from build123d import *

# Parameters (mm, degrees)
ESQUISSE1_W             = 15
ESQUISSE1_H             = 9.5
BOSS_EXTRU_1_DEPTH      = 0.3
ESQUISSE2_W             = 5
ESQUISSE2_H             = 5
BOSS_EXTRU_2_DEPTH      = 1.6
ESQUISSE3_R             = 2
ENL_V_MAT_EXTRU_1_DEPTH = 0.3
BOSS_EXTRU_3_DEPTH      = 0.2
CONG_1_R                = 0.5
ENL_V_MAT_EXTRU_2_DEPTH = 0.05
ESQUISSE6_W             = 1
ESQUISSE6_H             = 2
BOSS_EXTRU_4_DEPTH      = 1


with BuildPart() as part:
    # Esquisse1 → Boss.-Extru.1 (new body)
    with BuildSketch(Plane.XY):
        with Locations((7.5, 4.75)):
            Rectangle(ESQUISSE1_W, ESQUISSE1_H)
    extrude(amount=BOSS_EXTRU_1_DEPTH)

    # Esquisse2 → Boss.-Extru.2 (add)
    with BuildSketch(Plane.XY.offset(0.3)):
        with Locations((7.5, 4.75)):
            Rectangle(ESQUISSE2_W, ESQUISSE2_H)
    extrude(amount=BOSS_EXTRU_2_DEPTH)

    # Esquisse3 → Enlèv. mat.-Extru.1 (cut)
    with BuildSketch(Plane.XY.offset(1.9)):
        with Locations((7.5, 4.75)):
            Circle(ESQUISSE3_R)
        Polygon((9.292893219, 7.25), (10, 6.542893219), (10, 7.25), align=None)
    extrude(amount=-ENL_V_MAT_EXTRU_1_DEPTH, mode=Mode.SUBTRACT)

    # Esquisse4 → Boss.-Extru.3 (add)
    with BuildSketch(Plane.XY.offset(0.3)):
        with BuildLine():
            Line((8.875, 8.263238259), (8.625, 8.263238259))
            ThreePointArc((8.625, 8.263238259), (8.271446609, 8.11679165), (8.125, 7.763238259))
            Line((8.125, 7.763238259), (8.125, 7.25))
            Line((8.125, 7.25), (9.375, 7.25))
            Line((9.375, 7.25), (9.375, 7.763238259))
            ThreePointArc((9.375, 7.763238259), (9.228553391, 8.11679165), (8.875, 8.263238259))
        make_face()
        with BuildLine():
            Line((5.625, 7.25), (6.875, 7.25))
            Line((6.875, 7.25), (6.875, 7.763238259))
            ThreePointArc((6.875, 7.763238259), (6.728553391, 8.11679165), (6.375, 8.263238259))
            Line((6.375, 8.263238259), (6.125, 8.263238259))
            ThreePointArc((6.125, 8.263238259), (5.771446609, 8.11679165), (5.625, 7.763238259))
            Line((5.625, 7.763238259), (5.625, 7.25))
        make_face()
        with BuildLine():
            Line((9.375, 2.25), (9.375, 1.736761741))
            ThreePointArc((9.375, 1.736761741), (9.228553391, 1.38320835), (8.875, 1.236761741))
            Line((8.875, 1.236761741), (8.625, 1.236761741))
            ThreePointArc((8.625, 1.236761741), (8.271446609, 1.38320835), (8.125, 1.736761741))
            Line((8.125, 1.736761741), (8.125, 2.25))
            Line((8.125, 2.25), (9.375, 2.25))
        make_face()
        with BuildLine():
            Line((6.125, 1.236761741), (6.375, 1.236761741))
            ThreePointArc((6.375, 1.236761741), (6.728553391, 1.38320835), (6.875, 1.736761741))
            Line((6.875, 1.736761741), (6.875, 2.25))
            Line((6.875, 2.25), (5.625, 2.25))
            Line((5.625, 2.25), (5.625, 1.736761741))
            ThreePointArc((5.625, 1.736761741), (5.771446609, 1.38320835), (6.125, 1.236761741))
        make_face()
    extrude(amount=BOSS_EXTRU_3_DEPTH)

    # Congé1
    # the kernel refuses this fillet: 0.5 mm, written as the material it takes off along each edge
    with BuildSketch(Plane(origin=(8.125, 1.736761741, 0.5), x_dir=(2.6165736243852198e-11, 0, -1.0), z_dir=(0, 1, 0)), Plane(origin=(9.375, 2.25, 0.5), x_dir=(-2.6165736243852198e-11, 0, -1.0), z_dir=(0, -1, 0))) as cong_1_piece_1:
        with BuildLine():
            CenterArc((0.5, -0.4), CONG_1_R, 126.869897647, 53.130102355)
            Line((0, -0.4), (-0.01, -0.4))
            Line((-0.01, -0.4), (-0.01, 0))
            Line((-0.01, 0), (0, 0.01))
            ThreePointArc((0, 0.01), (0.1, 0.01), (0.194, 0.008))
            Line((0.194, 0.008), (0.2, 0))
        make_face()
    extrude(amount=0.513238259, mode=Mode.SUBTRACT)
    with BuildSketch(Plane(origin=(8.625, 1.736761741, 0.5), x_dir=(0, -1, 0), z_dir=(1, 0, 0))) as cong_1_piece_2:
        with BuildLine():
            CenterArc((0.1, 0.5), CONG_1_R, 270, 53.130102355)
            Line((0.1, 0), (0.1, -0.01))
            Line((0.1, -0.01), (0.5, -0.01))
            Line((0.5, -0.01), (0.51, 0))
            ThreePointArc((0.51, 0), (0.51, 0.1), (0.508, 0.194))
            Line((0.508, 0.194), (0.5, 0.2))
        make_face()
    revolve(axis=Axis((8.625, 1.736761741, 0.5), (0, 0, -1)), revolution_arc=90, mode=Mode.SUBTRACT)
    with BuildSketch(Plane(origin=(8.875, 1.236761741, 0.5), x_dir=(0, 2.6109114869598534e-11, -1.0), z_dir=(-1, 0, 0))) as cong_1_piece_3:
        with BuildLine():
            CenterArc((0.5, -0.4), CONG_1_R, 126.869897647, 53.130102355)
            Line((0, -0.4), (-0.01, -0.4))
            Line((-0.01, -0.4), (-0.01, 0))
            Line((-0.01, 0), (0, 0.01))
            ThreePointArc((0, 0.01), (0.1, 0.01), (0.194, 0.008))
            Line((0.194, 0.008), (0.2, 0))
        make_face()
    extrude(amount=0.25, mode=Mode.SUBTRACT)
    with BuildSketch(Plane(origin=(5.625, 2.25, 0.5), x_dir=(2.6059154833492393e-11, 0, -1.0), z_dir=(0, -1, 0)), Plane(origin=(6.875, 1.736761741, 0.5), x_dir=(-2.6112445538672294e-11, 0, -1.0), z_dir=(0, 1, 0)), Plane(origin=(6.875, 7.25, 0.5), x_dir=(-2.6112445538672294e-11, 0, -1.0), z_dir=(0, 1, 0)), Plane(origin=(5.625, 7.763238259, 0.5), x_dir=(2.6059154833492393e-11, 0, -1.0), z_dir=(0, -1, 0)), Plane(origin=(9.375, 7.25, 0.5), x_dir=(-2.6165736243852198e-11, 0, -1.0), z_dir=(0, 1, 0)), Plane(origin=(8.125, 7.763238259, 0.5), x_dir=(2.6165736243852198e-11, 0, -1.0), z_dir=(0, -1, 0))) as cong_1_piece_4:
        with BuildLine():
            CenterArc((0.5, 0.4), CONG_1_R, 179.999999999, 53.130102355)
            Line((0, 0.4), (-0.01, 0.4))
            Line((-0.01, 0.4), (-0.01, 0))
            Line((-0.01, 0), (0, -0.01))
            ThreePointArc((0, -0.01), (0.1, -0.01), (0.194, -0.008))
            Line((0.194, -0.008), (0.2, 0))
        make_face()
    extrude(amount=0.513238259, mode=Mode.SUBTRACT)
    with BuildSketch(Plane(origin=(6.125, 1.736761741, 0.5), x_dir=(-1, 0, 0), z_dir=(0, 1, 0))) as cong_1_piece_5:
        with BuildLine():
            CenterArc((0.1, -0.5), CONG_1_R, 36.869897645, 53.130102355)
            Line((0.1, 0), (0.1, 0.01))
            Line((0.1, 0.01), (0.5, 0.01))
            Line((0.5, 0.01), (0.51, 0))
            ThreePointArc((0.51, 0), (0.51, -0.1), (0.508, -0.194))
            Line((0.508, -0.194), (0.5, -0.2))
        make_face()
    revolve(axis=Axis((6.125, 1.736761741, 0.5), (0, 0, 1)), revolution_arc=90, mode=Mode.SUBTRACT)
    with BuildSketch(Plane(origin=(6.125, 1.236761741, 0.5), x_dir=(0, 2.6109114869598534e-11, -1.0), z_dir=(1, 0, 0)), Plane(origin=(6.375, 8.263238259, 0.5), x_dir=(0, -2.6112445538672342e-11, -1.0), z_dir=(-1, 0, 0)), Plane(origin=(8.875, 8.263238259, 0.5), x_dir=(0, -2.6112445538672342e-11, -1.0), z_dir=(-1, 0, 0))) as cong_1_piece_6:
        with BuildLine():
            CenterArc((0.5, 0.4), CONG_1_R, 179.999999999, 53.130102355)
            Line((0, 0.4), (-0.01, 0.4))
            Line((-0.01, 0.4), (-0.01, 0))
            Line((-0.01, 0), (0, -0.01))
            ThreePointArc((0, -0.01), (0.1, -0.01), (0.194, -0.008))
            Line((0.194, -0.008), (0.2, 0))
        make_face()
    extrude(amount=0.25, mode=Mode.SUBTRACT)
    with BuildSketch(Plane(origin=(6.125, 7.763238259, 0.5), x_dir=(0, 1, 0), z_dir=(1, 0, 0))) as cong_1_piece_7:
        with BuildLine():
            CenterArc((0.1, -0.5), CONG_1_R, 36.869897645, 53.130102355)
            Line((0.1, 0), (0.1, 0.01))
            Line((0.1, 0.01), (0.5, 0.01))
            Line((0.5, 0.01), (0.51, 0))
            ThreePointArc((0.51, 0), (0.51, -0.1), (0.508, -0.194))
            Line((0.508, -0.194), (0.5, -0.2))
        make_face()
    revolve(axis=Axis((6.125, 7.763238259, 0.5), (0, 0, 1)), revolution_arc=90, mode=Mode.SUBTRACT)
    with BuildSketch(Plane(origin=(8.875, 7.763238259, 0.5), x_dir=(1, 0, 0), z_dir=(0, -1, 0))) as cong_1_piece_8:
        with BuildLine():
            CenterArc((0.1, -0.5), CONG_1_R, 36.869897645, 53.130102355)
            Line((0.1, 0), (0.1, 0.01))
            Line((0.1, 0.01), (0.5, 0.01))
            Line((0.5, 0.01), (0.51, 0))
            ThreePointArc((0.51, 0), (0.51, -0.1), (0.508, -0.194))
            Line((0.508, -0.194), (0.5, -0.2))
        make_face()
    revolve(axis=Axis((8.875, 7.763238259, 0.5), (0, 0, 1)), revolution_arc=90, mode=Mode.SUBTRACT)
    with BuildSketch(Plane(origin=(8.875, 1.736761741, 0.5), x_dir=(1, 0, 0), z_dir=(0, 1, 0))) as cong_1_piece_9:
        with BuildLine():
            CenterArc((0.1, 0.5), CONG_1_R, 270, 53.130102355)
            Line((0.1, 0), (0.1, -0.01))
            Line((0.1, -0.01), (0.5, -0.01))
            Line((0.5, -0.01), (0.51, 0))
            ThreePointArc((0.51, 0), (0.51, 0.1), (0.508, 0.194))
            Line((0.508, 0.194), (0.5, 0.2))
        make_face()
    revolve(axis=Axis((8.875, 1.736761741, 0.5), (0, 0, -1)), revolution_arc=90, mode=Mode.SUBTRACT)
    with BuildSketch(Plane(origin=(6.375, 1.736761741, 0.5), x_dir=(0, -1, 0), z_dir=(-1, 0, 0))) as cong_1_piece_10:
        with BuildLine():
            CenterArc((0.1, -0.5), CONG_1_R, 36.869897645, 53.130102355)
            Line((0.1, 0), (0.1, 0.01))
            Line((0.1, 0.01), (0.5, 0.01))
            Line((0.5, 0.01), (0.51, 0))
            ThreePointArc((0.51, 0), (0.51, -0.1), (0.508, -0.194))
            Line((0.508, -0.194), (0.5, -0.2))
        make_face()
    revolve(axis=Axis((6.375, 1.736761741, 0.5), (0, 0, 1)), revolution_arc=90, mode=Mode.SUBTRACT)
    with BuildSketch(Plane(origin=(6.375, 7.763238259, 0.5), x_dir=(1, 0, 0), z_dir=(0, -1, 0))) as cong_1_piece_11:
        with BuildLine():
            CenterArc((0.1, -0.5), CONG_1_R, 36.869897645, 53.130102355)
            Line((0.1, 0), (0.1, 0.01))
            Line((0.1, 0.01), (0.5, 0.01))
            Line((0.5, 0.01), (0.51, 0))
            ThreePointArc((0.51, 0), (0.51, -0.1), (0.508, -0.194))
            Line((0.508, -0.194), (0.5, -0.2))
        make_face()
    revolve(axis=Axis((6.375, 7.763238259, 0.5), (0, 0, 1)), revolution_arc=90, mode=Mode.SUBTRACT)
    with BuildSketch(Plane(origin=(8.625, 7.763238259, 0.5), x_dir=(0, 1, 0), z_dir=(1, 0, 0))) as cong_1_piece_12:
        with BuildLine():
            CenterArc((0.1, -0.5), CONG_1_R, 36.869897645, 53.130102355)
            Line((0.1, 0), (0.1, 0.01))
            Line((0.1, 0.01), (0.5, 0.01))
            Line((0.5, 0.01), (0.51, 0))
            ThreePointArc((0.51, 0), (0.51, -0.1), (0.508, -0.194))
            Line((0.508, -0.194), (0.5, -0.2))
        make_face()
    revolve(axis=Axis((8.625, 7.763238259, 0.5), (0, 0, 1)), revolution_arc=90, mode=Mode.SUBTRACT)

    # Esquisse5 → Enlèv. mat.-Extru.2 (cut)
    with BuildSketch(Plane.XY.offset(0.3)):
        with BuildLine():
            Line((-1.5, 1.525), (0.7, 1.525))
            ThreePointArc((0.7, 1.525), (1.265685425, 1.759314575), (1.5, 2.325))
            Line((1.5, 2.325), (1.5, 2.425))
            ThreePointArc((1.5, 2.425), (1.265685425, 2.990685425), (0.7, 3.225))
            Line((0.7, 3.225), (-1.5, 3.225))
            Line((-1.5, 3.225), (-1.5, 1.525))
        make_face()
        with BuildLine():
            Line((-1.5, 3.9), (0.7, 3.9))
            ThreePointArc((0.7, 3.9), (1.265685425, 4.134314575), (1.5, 4.7))
            Line((1.5, 4.7), (1.5, 4.8))
            ThreePointArc((1.5, 4.8), (1.265685425, 5.365685425), (0.7, 5.6))
            Line((0.7, 5.6), (-1.5, 5.6))
            Line((-1.5, 5.6), (-1.5, 3.9))
        make_face()
        with BuildLine():
            Line((-1.5, 6.275), (0.7, 6.275))
            ThreePointArc((0.7, 6.275), (1.265685425, 6.509314575), (1.5, 7.075))
            Line((1.5, 7.075), (1.5, 7.175))
            ThreePointArc((1.5, 7.175), (1.265685425, 7.740685425), (0.7, 7.975))
            Line((0.7, 7.975), (-1.5, 7.975))
            Line((-1.5, 7.975), (-1.5, 6.275))
        make_face()
        with BuildLine():
            Line((16.5, 3.225), (16.5, 1.525))
            Line((16.5, 1.525), (14.3, 1.525))
            ThreePointArc((14.3, 1.525), (13.734314575, 1.759314575), (13.5, 2.325))
            Line((13.5, 2.325), (13.5, 2.425))
            ThreePointArc((13.5, 2.425), (13.734314575, 2.990685425), (14.3, 3.225))
            Line((14.3, 3.225), (16.5, 3.225))
        make_face()
        with BuildLine():
            Line((16.5, 5.6), (14.3, 5.6))
            ThreePointArc((14.3, 5.6), (13.734314575, 5.365685425), (13.5, 4.8))
            Line((13.5, 4.8), (13.5, 4.7))
            ThreePointArc((13.5, 4.7), (13.734314575, 4.134314575), (14.3, 3.9))
            Line((14.3, 3.9), (16.5, 3.9))
            Line((16.5, 3.9), (16.5, 5.6))
        make_face()
        with BuildLine():
            Line((16.5, 7.975), (14.3, 7.975))
            ThreePointArc((14.3, 7.975), (13.734314575, 7.740685425), (13.5, 7.175))
            Line((13.5, 7.175), (13.5, 7.075))
            ThreePointArc((13.5, 7.075), (13.734314575, 6.509314575), (14.3, 6.275))
            Line((14.3, 6.275), (16.5, 6.275))
            Line((16.5, 6.275), (16.5, 7.975))
        make_face()
    extrude(amount=-ENL_V_MAT_EXTRU_2_DEPTH, mode=Mode.SUBTRACT)

    # Esquisse6 → Boss.-Extru.4 (add)
    with BuildSketch(Plane.XY.offset(0.3)):
        with Locations((11.04087009, 4.75)):
            Rectangle(ESQUISSE6_W, ESQUISSE6_H)
    extrude(amount=BOSS_EXTRU_4_DEPTH)


solid = part.part
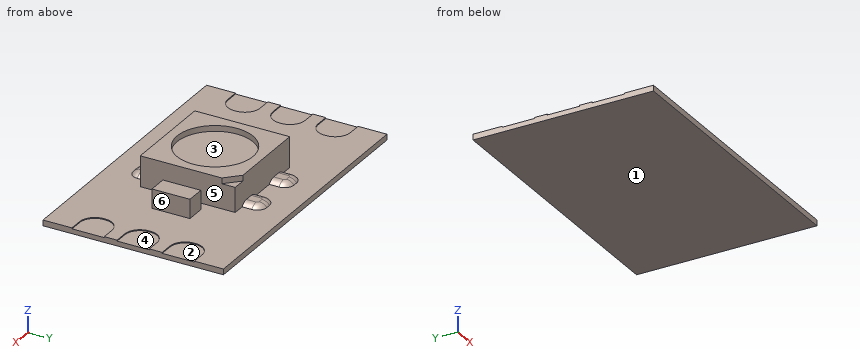
Design review of the part built by this model. Coordinates are the model's own, in mm. Face numbers are marked on the shaded views. A direction names the side the tool comes from. Give positions to 0.01 mm unless a question says otherwise; leave off trailing zeros. Loops run counter-clockwise (first coordinate to the right, second up) from the corner with the lowest first, then second, coordinate; pieces in that order, holes last. Notation, with made-up numbers: M 2,-15 L 29,-15 A29 cw 29,14 Z; hole C 19,68.5 d11. An arc over 180 degrees is marked long. One line per question, with ' | ' between items. Start each with the question number.
1. Add section D-D (y = 1). Write out the cut boundary in (x, z).
2. For the marked faces 1, 2 and 3, list the 3-axis set-ups (+Z, -Z, +X, -X, +Y, -Y) from which the entire face can be reached by the end or side of a thin tool; tool diameter is ignored.
3. The part is to be moulded in two halves that separate along X. For the marked faces 4, 5 and 6, say which applies: released by +X, released by -X, zero draft, split by the parting line, or undercut.
4. To check wall thickness, follow L1, parallel to Y at x = 7.5, z = 1.8; L2, parallel to X at y = 4.75, z = 0.7; L3, parallel to Z at x = 8.5, y = 5.5. State the ranges of each line that lie inside material, in increasing order.
5. Insertion check: P1, Ø1, axis at y = 5, z = 1.5, coming from the +X side; P2, Ø1.2, axis at x = 8, y = 5.5, coming from the +Z side. Each pin has a flat end and moves straight along its axis. Give the tip position at first contact, or say it passes through.
6. Add section C-C (x = 7.5). Write out the cut boundary in (y, z), plus the area to 3 significant figures.
7. Add section B-B (z = 1.75). Write out the cut boundary in (x, y).
8. Add section A-A (z = 0.85). Write out the cut boundary in (x, y).
Worked out:
1) outline: M 0,0 L 15,0 L 15,0.3 L 0,0.3 Z
2) face 1: -Z, +X, -X, +Y, -Y | face 2: +Z, +X | face 3: +Z
3) face 4: zero draft | face 5: undercut | face 6: released by +X
4) L1: y = 2.25 to 2.75, 6.75 to 7.25 | L2: x = 5 to 10, 10.54 to 11.54 | L3: z = 0 to 1.6
5) P1: stops at x = 11.54 | P2: stops at z = 1.6
6) outline: M 0,0 L 9.5,0 L 9.5,0.3 L 7.25,0.3 L 7.25,1.9 L 6.75,1.9 L 6.75,1.6 L 2.75,1.6 L 2.75,1.9 L 2.25,1.9 L 2.25,0.3 L 0,0.3 Z | area: 9.65 mm²
7) outline: M 5,2.25 L 10,2.25 L 10,6.54 L 9.29,7.25 L 5,7.25 Z; hole C 7.5,4.75 d4
8) outline: M 5,2.25 L 10,2.25 L 10,7.25 L 5,7.25 Z; M 10.54,3.75 L 11.54,3.75 L 11.54,5.75 L 10.54,5.75 Z
